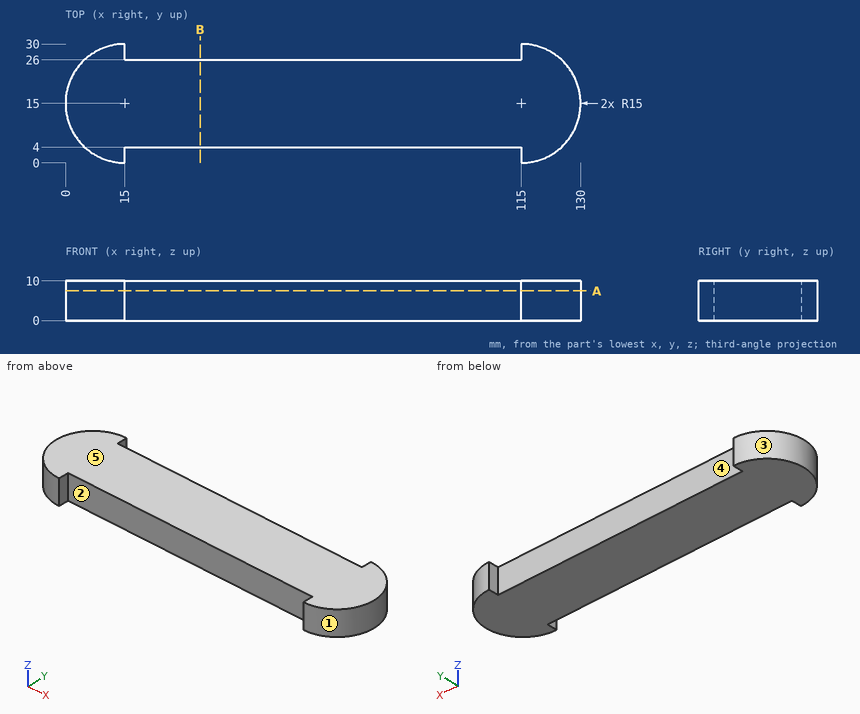
Geometry: see drawing. Coordinates: mm, zero at the bounding-box minimum. A direction names the side the tool comes from. Give positions to 0.01 mm unless a question says otherwise; leave off trailing zeros. Loops run counter-clockwise (first coordinate to the right, second up) from the corner with the lowest first, then second, coordinate; pieces in that order, holes last. Notation, with made-up numbers: (65.5, 74.5) - (122.5, 74.5) arc R20 cw to (122.5, 112.5) - close; hole circle Ø4 at (81.5, 15.25). An arc over 180 degrees is marked (long way). Answer as CSV lines item,"result". Start each with the question number.
1. Draft query along X for the marked faces 1, 2 and 3. Return one class per face: released by +X, released by -X, zero draft, split by the parting line, or undercut.
2. Section B-B, the plane x = 34. Return loops of the section in (y, z).
3. Pin query (flat end, axial travel): P1, Ø1, axis at y = 3, z = 2, coming from the -X side; P2, Ø3, axis at y = 21, z = 3, coming from the +X side; P3, Ø6, axis at x = 47.5, z = 1.5, coming from the +Y side. Return the tip coordinate at first contact, or that it passes through.
4. Section A-A, the plane z = 7.5. Return loops of the section in (x, y), plus the area to 3 significant figures.
5. Ray query, L1, parallel to Y at x = 94, z = 3.75; L2, parallel to X at y = 2.75, z = 6.5; L3, parallel to X at y = 26.5, z = 7.75. Return the intervals inside material, ascending.
6. Reachability of the marked faces 4 and 5 from +Z, -Z, +X, -X, +Y, -Y: full face, straight path, thin tool, end or side. Return the list, or none.
Answers:
1,face 1,"released by +X"
1,face 2,"undercut"
1,face 3,"released by -X"
2,outline,"(4, 0) - (26, 0) - (26, 10) - (4, 10) - close"
3,P1,"stops at x = 5.37"
3,P2,"stops at x = 129.31"
3,P3,"stops at y = 26"
4,outline,"(15, 0) - (15, 4) - (115, 4) - (115, 0) arc R15 ccw to (115, 30) - (115, 26) - (15, 26) - (15, 30) arc R15 ccw to start"
4,area,"2,910 mm2"
5,L1,"y = 4 to 26"
5,L2,"x = 6.34 to 15, 115 to 123.66"
5,L3,"x = 5.37 to 15, 115 to 124.63"
6,face 4,"+Z, -Z, +Y"
6,face 5,"+Z, +X, -X, +Y, -Y"
